For this review, take the finished solid that the model builds, in its own axes (mm). Give positions to 0.01 mm unless a question says otherwise; leave off trailing zeros. Order: outer loops, then holes, each group sorted by start corner. A loop starts at its lowest first (then second) coordinate and runs counter-clockwise, first axis right, second up.
from build123d import *

# Parameters (mm, degrees)
F0_W     = 100
F0_H     = 50
F1_DEPTH = 50
F2_R     = 9.118909
F3_DEPTH = 50
F4_R     = 10.179687
F5_DEPTH = 50


with BuildPart() as f1:
    # F0 (on Top) → F1 (new body)
    with BuildSketch(Plane.XY):
        with Locations((-2.810752, -6.296756)):
            Rectangle(F0_W, F0_H)
    extrude(amount=F1_DEPTH)

    # F2 (on face) → F3 (cut, through all)
    with BuildSketch(Plane.XY.offset(50)):
        with Locations((-8.071532, -15.383557)):
            Circle(F2_R)
    extrude(amount=-F3_DEPTH, mode=Mode.SUBTRACT)

    # F4 (on face) → F5 (cut, through all)
    with BuildSketch(Plane(origin=(0, 18.703244, 0), x_dir=(-1, 0, 0), z_dir=(0, 1, 0))):
        with Locations((28.091645, 28.360171)):
            Circle(F4_R)
    extrude(amount=-F5_DEPTH, mode=Mode.SUBTRACT)


solid = f1.part
1) We need section B-B on z = 26. Give the boundary of the cut face in (x, y), then the cut area to 3 significant figures.
Answer sheet:
outline: (-52.81, -31.3) - (-37.99, -31.3) - (-37.99, 18.7) - (-52.81, 18.7) - close; (-18.19, -31.3) - (47.19, -31.3) - (47.19, 18.7) - (-18.19, 18.7) - close; hole circle Ø18.24 at (-8.07, -15.38)
area: 3,750 mm2
2) Draft analysis for pull direction X (two halves, no side actions). For faces 1 (the face through (47.189, -7, 25)), 2 (the face through (-3.86, -23.47, 25.35)), 3 (the face through (-4, -6, 50)), state which applies: +X half, -X half, draft (parallel to the pull), parting line (faces both ways), or undercut.
Answer sheet:
face 1: +X half
face 2: undercut
face 3: draft
3) We need section C-C on x = -24. Give the boundary of the cut face in (y, z).
Answer sheet:
outline: (-31.3, 0) - (18.7, 0) - (18.7, 19.04) - (-31.3, 19.04) - close; (-31.3, 37.68) - (18.7, 37.68) - (18.7, 50) - (-31.3, 50) - close
4) We need section A-A on y = -9.5. Give the boundary of the cut face in (x, z), then the cut area to 3 significant figures.
Answer sheet:
outline: (-52.81, 0) - (-15.04, 0) - (-15.04, 50) - (-52.81, 50) - close; (-1.1, 0) - (47.19, 0) - (47.19, 50) - (-1.1, 50) - close; hole circle Ø20.36 at (-28.09, 28.36)
area: 3,980 mm2
5) We need section D-D on z = 9.5. Give the boundary of the cut face in (x, y).
Answer sheet:
outline: (-52.81, -31.3) - (47.19, -31.3) - (47.19, 18.7) - (-52.81, 18.7) - close; hole circle Ø18.24 at (-8.07, -15.38)
6) To check wall thickness, follow line 1 (X direction, y = -13, z = 29); line 2 (Z direction, x = -28, y = 12); line 3 (X direction, y = -22, z = 28.5). State the ranges of each line that lie inside material, in increasing order.
Answer sheet:
line 1: x = -52.81 to -38.25, -17.93 to -16.87, 0.73 to 47.19
line 2: z = 0 to 18.18, 38.54 to 50
line 3: x = -52.81 to -38.27, -17.91 to -14.35, -1.8 to 47.19
